Source: CAD feature listing. Evaluate the final solid. Frame: model axes, mm. Face numbers are marked on the shaded views. A direction names the side the tool comes from. Give positions to 0.01 mm unless a question says otherwise; leave off trailing zeros. Loops run counter-clockwise (first coordinate to the right, second up) from the corner with the lowest first, then second, coordinate; pieces in that order, holes last.
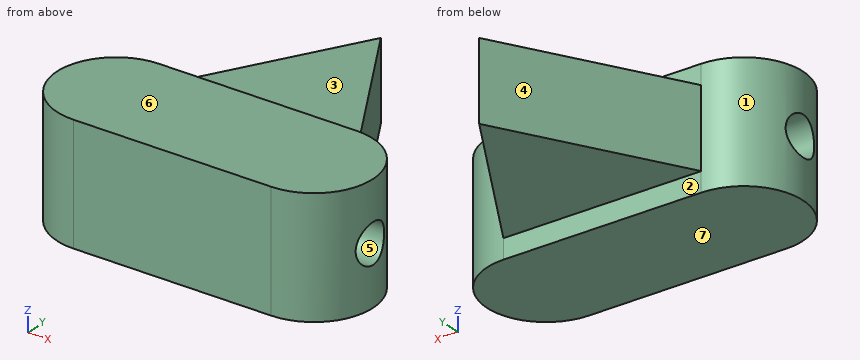
```python
from build123d import *

# Parameters (mm, degrees)
SKETCH3_W               = 127
SKETCH3_H               = 76.2
BOSS_EXTRUDE1_DEPTH     = 76.2
BOSS_EXTRUDE2_DEPTH     = 76.2
BOSS_EXTRUDE3_DEPTH     = 25.4
SKETCH6_R               = 12.7
CUT_EXTRUDE1_DEPTH      = 102.6
CUT_EXTRUDE1_DEPTH_BACK = 102.6


with BuildPart() as part:
    # Sketch3 → Boss-Extrude1 (new body)
    with BuildSketch(Plane(origin=(0, 0, 0), x_dir=(1, 0, 0), z_dir=(0, 1, 0))):
        Rectangle(SKETCH3_W, SKETCH3_H)
    extrude(amount=BOSS_EXTRUDE1_DEPTH)

    # Sketch4 → Boss-Extrude2 (add)
    with BuildSketch(Plane.XY.offset(38.1)):
        with BuildLine():
            Line((-63.5, 76.2), (-63.5, 0))
            ThreePointArc((-63.5, 0), (-101.6, 38.1), (-63.5, 76.2))
        make_face()
        with BuildLine():
            Line((63.5, 76.2), (63.5, 0))
            ThreePointArc((63.5, 0), (101.6, 38.1), (63.5, 76.2))
        make_face()
    extrude(amount=-BOSS_EXTRUDE2_DEPTH)

    # Sketch5 → Boss-Extrude3 (add, symmetric)
    with BuildSketch(Plane.XY):
        Polygon((-63.5, 76.2), (63.5, 76.2), (0, 186.185226281), align=None)
    extrude(amount=BOSS_EXTRUDE3_DEPTH, both=True)

    # Sketch6 → Cut-Extrude1 (cut, two sides)
    with BuildSketch(Plane(origin=(0, 0, 0), x_dir=(0, 0, -1), z_dir=(1, 0, 0))) as cut_extrude1_sk:
        with Locations((0, 38.1)):
            Circle(SKETCH6_R)
    extrude(amount=CUT_EXTRUDE1_DEPTH, mode=Mode.SUBTRACT)
    extrude(cut_extrude1_sk.sketch, amount=-CUT_EXTRUDE1_DEPTH_BACK, mode=Mode.SUBTRACT)


solid = part.part
```
(1) Mould query, pull axis Z, two halves, no side actions, for the marked faces 4, 5, 6 and 7. Classes: pulls with the +Z half, pulls with the -Z half, needs draft (parallel to the pull), parting line crosses it, or undercut.
A:
face 4: needs draft
face 5: undercut
face 6: pulls with the +Z half
face 7: pulls with the -Z half
(2) Reachability of the marked faces 1, 2 and 3 from +Z, -Z, +X, -X, +Y, -Y: full face, straight path, thin tool, end or side. Return the list, or none.
A:
face 1: +Z, -Z, -X
face 2: -Z, +X, -X, +Y
face 3: +Z, +X, -X, +Y
(3) Section C-C, the plane x = 6. Return the cut outline in (y, z), then the cut area to 3 significant figures.
A:
outline: (0, -38.1) - (76.2, -38.1) - (76.2, -25.4) - (175.79, -25.4) - (175.79, 25.4) - (76.2, 25.4) - (76.2, 38.1) - (0, 38.1) - close; hole circle Ø25.4 at (38.1, 0)
area: 10,400 mm2
(4) Section A-A, the plane y = 38.1. Return the cut outline in (x, z).
A:
outline: (-101.6, -38.1) - (101.6, -38.1) - (101.6, -12.7) - (-101.6, -12.7) - close; (-101.6, 12.7) - (101.6, 12.7) - (101.6, 38.1) - (-101.6, 38.1) - close
(5) Section B-B, the plane z = 0. Return the cut outline in (x, y).
A:
outline: (-99.42, 25.4) arc R38.1 ccw to (-63.5, 0) - (63.5, 0) arc R38.1 ccw to (99.42, 25.4) - close; (-99.42, 50.8) - (99.42, 50.8) arc R38.1 ccw to (63.5, 76.2) - (0, 186.19) - (-63.5, 76.2) arc R38.1 ccw to start
(6) First-contact query: pin 1 (12 mm diameter, centred on x = 14, z = -12.5, fed in from +Y); pin 2 (3 mm diameter, centred on y = 23.5, z = -13.5, fed in from +X); pin 3 (6 mm diameter, centred on x = -6, z = 27, fed in from +Y). Flat tips, straight axial feed; report the tip coordinate or a pass-through.
A:
pin 1: stops at y = 172.33
pin 2: stops at x = 99.28
pin 3: stops at y = 180.19
(7) Ray query, line 1 along Z through (x, y) = (30, 38); line 2 along Y through (x, z) = (-23.5, 27.5); line 3 along Y through (x, z) = (-74.5, -11.5). Return the intervals inside material, ascending.
A:
line 1: z = -38.1 to -12.7, 12.7 to 38.1
line 2: y = 0 to 76.2
line 3: y = 1.62 to 32.71, 43.49 to 74.58
(8) Section D-D, the plane z = -30. Return the cut outline in (x, y).
A:
outline: (-63.5, 0) - (63.5, 0) arc R38.1 ccw to (63.5, 76.2) - (-63.5, 76.2) arc R38.1 ccw to start
